from build123d import *

# Parameters (mm, degrees)
SKETCH1_W           = 225
SKETCH1_H           = 115
BOSS_EXTRUDE1_DEPTH = 4
SKETCH3_R           = 2.5
SKETCH3_W           = 5.58
SKETCH3_H           = 5
CUT_EXTRUDE2_DEPTH  = 10
SKETCH4_W           = 4
SKETCH4_H           = 39
BOSS_EXTRUDE2_DEPTH = 4
SKETCH5_W           = 45
SKETCH5_H           = 4
BOSS_EXTRUDE3_DEPTH = 4
LPATTERN1_COUNT     = 2
LPATTERN1_PITCH     = 229
SKETCH6_W           = 23
SKETCH6_H           = 4
BOSS_EXTRUDE4_DEPTH = 4
SKETCH7_W           = 32
SKETCH7_H           = 4
BOSS_EXTRUDE5_DEPTH = 4
SKETCH8_W           = 4
SKETCH8_H           = 2
BOSS_EXTRUDE6_DEPTH = 4


with BuildPart() as part:
    # Sketch1 → Boss-Extrude1 (new body)
    with BuildSketch(Plane(origin=(0, 0, 0), x_dir=(1, 0, 0), z_dir=(0, 1, 0))):
        with Locations((112.5, 57.5)):
            Rectangle(SKETCH1_W, SKETCH1_H)
    extrude(amount=BOSS_EXTRUDE1_DEPTH)

    # Sketch3 → Cut-Extrude2 (cut)
    with BuildSketch(Plane(origin=(0, 4, 0), x_dir=(1, 0, 0), z_dir=(0, 1, 0))):
        with Locations(Location((180.08999958, 22.78, 0), (0, 0, 270))):
            Circle(SKETCH3_R)
        with Locations(Location((172.08999958, 22.78, 0), (0, 0, 270))):
            Circle(SKETCH3_R)
        with Locations(Location((164.08999958, 22.78, 0), (0, 0, 270))):
            Circle(SKETCH3_R)
        with Locations((149.29999958, 22.78)):
            Rectangle(SKETCH3_W, SKETCH3_H)
        with Locations(Location((180.08999958, 48.49, 0), (0, 0, 270))):
            Circle(SKETCH3_R)
        with Locations(Location((172.08999958, 48.49, 0), (0, 0, 270))):
            Circle(SKETCH3_R)
        with Locations(Location((164.08999958, 48.49, 0), (0, 0, 270))):
            Circle(SKETCH3_R)
        with Locations((149.29999958, 48.49)):
            Rectangle(SKETCH3_W, SKETCH3_H)
        with Locations(Location((180.08999958, 74.2, 0), (0, 0, 270))):
            Circle(SKETCH3_R)
        with Locations(Location((172.08999958, 74.2, 0), (0, 0, 270))):
            Circle(SKETCH3_R)
        with Locations(Location((164.08999958, 74.2, 0), (0, 0, 270))):
            Circle(SKETCH3_R)
        with Locations((149.29999958, 74.2)):
            Rectangle(SKETCH3_W, SKETCH3_H)
        with Locations((116.37999958, 74.2)):
            Rectangle(SKETCH3_W, SKETCH3_H)
        with Locations((116.37999958, 48.49)):
            Rectangle(SKETCH3_W, SKETCH3_H)
        with Locations((116.37999958, 22.78)):
            Rectangle(SKETCH3_W, SKETCH3_H)
        with Locations(Location((101.58999958, 22.78, 0), (0, 0, 270))):
            Circle(SKETCH3_R)
        with Locations(Location((93.58999958, 22.78, 0), (0, 0, 270))):
            Circle(SKETCH3_R)
        with Locations(Location((85.58999958, 22.78, 0), (0, 0, 270))):
            Circle(SKETCH3_R)
        with Locations(Location((85.58999958, 48.49, 0), (0, 0, 270))):
            Circle(SKETCH3_R)
        with Locations(Location((93.58999958, 48.49, 0), (0, 0, 270))):
            Circle(SKETCH3_R)
        with Locations(Location((101.58999958, 48.49, 0), (0, 0, 270))):
            Circle(SKETCH3_R)
        with Locations(Location((101.58999958, 74.2, 0), (0, 0, 270))):
            Circle(SKETCH3_R)
        with Locations(Location((93.58999958, 74.2, 0), (0, 0, 270))):
            Circle(SKETCH3_R)
        with Locations(Location((85.58999958, 74.2, 0), (0, 0, 270))):
            Circle(SKETCH3_R)
    extrude(amount=-CUT_EXTRUDE2_DEPTH, mode=Mode.SUBTRACT)

    # Sketch4 → Boss-Extrude2 (add)
    with BuildSketch(Plane(origin=(0, 4, 0), x_dir=(1, 0, 0), z_dir=(0, 1, 0))):
        with Locations((-2, 19.5)):
            Rectangle(SKETCH4_W, SKETCH4_H)
        with Locations((-2, 97.5)):
            Rectangle(SKETCH4_W, SKETCH4_H)
    boss_extrude2 = extrude(amount=-BOSS_EXTRUDE2_DEPTH)

    # Sketch5 → Boss-Extrude3 (add)
    with BuildSketch(Plane(origin=(0, 4, 0), x_dir=(1, 0, 0), z_dir=(0, 1, 0))):
        with Locations((112.5, 117)):
            Rectangle(SKETCH5_W, SKETCH5_H)
        with Locations((202.5, 117)):
            Rectangle(SKETCH5_W, SKETCH5_H)
        with Locations((22.5, 117)):
            Rectangle(SKETCH5_W, SKETCH5_H)
    extrude(amount=-BOSS_EXTRUDE3_DEPTH)

    # LPattern1: Boss-Extrude2 ×2
    with Locations(*[(i * LPATTERN1_PITCH, 0, 0) for i in range(1, LPATTERN1_COUNT)]):
        add(boss_extrude2)

    # Sketch6 → Boss-Extrude4 (add)
    with BuildSketch(Plane(origin=(0, 4, 0), x_dir=(1, 0, 0), z_dir=(0, 1, 0))):
        with Locations((34.5, -2)):
            Rectangle(SKETCH6_W, SKETCH6_H)
    extrude(amount=-BOSS_EXTRUDE4_DEPTH)

    # Sketch7 → Boss-Extrude5 (add)
    with BuildSketch(Plane(origin=(0, 4, 0), x_dir=(1, 0, 0), z_dir=(0, 1, 0))):
        with Locations((181, -2)):
            Rectangle(SKETCH7_W, SKETCH7_H)
        with Locations((117, -2)):
            Rectangle(SKETCH7_W, SKETCH7_H)
    extrude(amount=-BOSS_EXTRUDE5_DEPTH)

    # Sketch8 → Boss-Extrude6 (add)
    with BuildSketch(Plane(origin=(0, 4, 0), x_dir=(1, 0, 0), z_dir=(0, 1, 0))):
        with Locations((-2, 118)):
            Rectangle(SKETCH8_W, SKETCH8_H)
        with Locations((227, 118)):
            Rectangle(SKETCH8_W, SKETCH8_H)
    extrude(amount=-BOSS_EXTRUDE6_DEPTH)


solid = part.part
Source: CAD feature listing. Evaluate the final solid. Frame: model axes, mm. A direction names the side the tool comes from. Give positions to 0.01 mm unless a question says otherwise; leave off trailing zeros. Write each loop counter-clockwise with the first axis right and the second up, starting at its lowest first coordinate (ties: lowest second). Pieces come first, ordered by that corner, then holes. Notation, with made-up numbers: M 32,53.25 L 51,53.25 A22 ccw 51,79.25 Z; hole C 20.25,62 d3. An arc over 180 degrees is marked long. Return JSON: item names as keys, results as strings. Group by question number.
1) Set-up query: faces 4 (the face through (73, 2, 0)), 5 (the face through (-2, 2, -78)), 6 (the face through (119.17, 2, -74)). Return all of +Z, -Z, +X, -X, +Y, -Y with unobstructed straight access to the full face (end or side cutting, diameter ignored); none if empty.
2) Pull-direction query (X, two-part tool) for faces 1 (the face through (229, 2, -98)), 2 (the face through (34, 2, 4)), 3 (the face through (99.37, 2.03, -47.34)); classes: pulls with the +X half, pulls with the -X half, needs draft (parallel to the pull), parting line crosses it, or undercut.
3) Cut plane D-D, the plane z = -69. Output: boundary loops of the cut face in (x, y), plus the area to 3 significant figures.
4) Material intervals for line 1 along Z through (x, y) = (101.59, 1.9); line 2 along Z through (x, y) = (93.59, 2.5); line 3 along Z through (x, y) = (17, 1.8), sorted ascending. Write a range as [from, to].
5) Cut plane A-A, the plane x = 85.59. Output: boundary loops of the cut face in (y, z), plus the area to 3 significant figures.
6) Cut plane B-B, the plane z = -22.78. Give the number of separate pieces and of enclosed holes in the cut face, plus the area to 3 significant figures.
7) Pin query (flat end, axial travel): P1, Ø2, axis at y = 1.5, z = -62.5, coming from the +X side; P2, Ø1.5, axis at x = 46, z = -82, coming from the -Y side; P3, Ø2, axis at y = 3, z = 2.5, coming from the +X side; P4, Ø4.5, axis at x = 85.59, z = -48.49, coming from the -Y side. Return the tip coordinate at first contact, or that it passes through.
Recorded:
{
 "1": {"face 4": "+Z, +Y, -Y", "face 5": "-X, +Y, -Y", "face 6": "+Y, -Y"},
 "2": {"face 1": "pulls with the +X half", "face 2": "needs draft", "face 3": "undercut"},
 "3": {"outline": "M 0,0 L 225,0 L 225,4 L 0,4 Z", "area": "900 mm²"},
 "4": {"line 1": "z = [-119, -76.7], [-71.7, -50.99], [-45.99, -25.28], [-20.28, 4]", "line 2": "z = [-119, -76.7], [-71.7, -50.99], [-45.99, -25.28], [-20.28, 0]", "line 3": "z = [-119, 0]"},
 "5": {"outline": "M 0,-115 L 4,-115 L 4,-76.7 L 0,-76.7 Z; M 0,-71.7 L 4,-71.7 L 4,-50.99 L 0,-50.99 Z; M 0,-45.99 L 4,-45.99 L 4,-25.28 L 0,-25.28 Z; M 0,-20.28 L 4,-20.28 L 4,0 L 0,0 Z", "area": "400 mm²"},
 "6": {"separate pieces": "9", "enclosed holes": "0", "area": "767 mm²"},
 "7": {"P1": "stops at x = 225", "P2": "stops at y = 0", "P3": "stops at x = 197", "P4": "passes through"}
}
